Autodesk Inventor part; units mm, degrees
ref_plane "Начальная плоскость" through (0, 0, -32.5) normal (0, 0, 1) x (1, 0, 0)
ref_plane "Конечная плоскость" through (0, 0, 510.459) normal (0, 0, 1) x (1, 0, 0)
ref_plane "РабПлоскость8" through (0, 0, 510.459) normal (0, 0, 1) x (1, 0, 0)
ref_plane "Начальная плоскость" through (0, 0, -32.5) normal (0, 0, 1) x (1, 0, 0)
ref_plane "Конечная плоскость" through (0, 0, 510.459) normal (0, 0, 1) x (1, 0, 0)
sketch "Эскиз" plane through (0, 0, 0) normal (0, 0, 1) x (1, 0, 0)
  line L0 (36, -32.5) -> (0, -32.5)
  line L1 (36, -32.5) -> (36, -28.696)
  line L2 (33.6994, -26.2039) -> (9.9215, -24.3017)
  line L3 (4.4, -18.3208) -> (4.4, 18.3208)
  line L4 (33.6994, 26.2039) -> (9.9215, 24.3017)
  line L5 (36, 28.696) -> (36, 32.5)
  line L6 (0, 32.5) -> (36, 32.5)
  line L7 (0, -32.5) -> (0, 32.5)
  arc A0 (4.4, -18.3208) -> (9.9215, -24.3017) centre (10.4, -18.3208) ccw
  arc A1 (9.9215, 24.3017) -> (4.4, 18.3208) centre (10.4, 18.3208) ccw
  arc A2 (36, -28.696) -> (33.6994, -26.2039) centre (33.5, -28.696) ccw
  arc A3 (33.6994, 26.2039) -> (36, 28.696) centre (33.5, 28.696) ccw
  line L8 (0, 45.5) -> (0, -45.5) construction
  line L9 (-7.2974, 0) -> (43.7847, 0) construction
  point P0 (36, -26.388)
  point P1 (4.4, -23.86)
  point P2 (4.4, 23.86)
  point P3 (36, 26.388)
  dimension "d3" = 36
  dimension "d5" = 4.4
  dimension "d7" = 65
  dimension "d9" = 8.64
  dimension "d11" = 8.64
  dimension "d13" = 6.112
  dimension "d15" = 6.112
  dimension "d22" = 6
  dimension "d23" = 2.5
  dimension "d24" = 32.5
  dimension "d25" = 0
extrude "Тело" add sketch "Эскиз" along normal up to surface (542.959 mm away) from surface at -32.5
sketch "Sketch3" plane through (0, 0, 0) normal (0, 0, 1) x (1, 0, 0)
  line L0 (0, 0) -> (10, 0)
ref_plane "Work Plane7" through (0, 0, 0) normal (0, -1, 0) x (1, 0, 0)
sketch "Sketch4" plane through (0, 0, 0) normal (0, -1, 0) x (1, 0, 0)
  line L0 (-2, -32.5) -> (12, -32.5)
  line L1 (-2, 510.459) -> (12, 510.459)
  dimension "d29" = 542.959
ref_plane "РабПлоскость8" through (0, 0, 510.459) normal (0, 0, 1) x (1, 0, 0)
split "Разделение1" plane through (0, 0, 510.459) removes the side toward (0, 0, 1)
ref_plane "РабПлоскость9" through (18, 177.5, -32.5) normal (0, 0, -1) x (-1, 0, 0)
split "Разделение2" plane through (18, 177.5, -32.5) removes the side toward (0, 0, -1)
equation "\"d3\" = b"
equation "\"d7\" = ParH"
equation "\"d22\" = R"
equation "\"d23\" = R1"
equation "\"d24\" = 0.5 * d7"
equation "\"d16\" = G_L"
equation "\"R1\" = 2.5"
equation "\"R\" = 6"
equation "\"t1\" = 4.4"
equation "\"t2\" = 7.2"
equation "\"ParH\" = 65"
equation "\"b\" = 36"
equation "\"msp_x1\" = 0.04 * b"
equation "\"msp_x2\" = -0.08 * t1 + 0.04 * b"
equation "\"G_L\" = d29"
equation "\"ex\" = 0"
equation "\"G_OFFSET_START\" = 32.5"
equation "\"G_OFFSET_END\" = -36"
equation "\"d26\" = -G_OFFSET_START"
equation "\"d27\" = G_OFFSET_END + B_L"
equation "\"B_L\" = 546.459"
properties part number "Швеллер 6.5U-542,96 ГОСТ 8240-97"
Geometry: final body of the model. Coordinates: model frame, mm. A direction names the side the tool comes from. Coordinates: 2 decimals unless noted, no trailing zeros. Order: outer loops, then holes, each group sorted by start corner. A loop starts at its lowest first (then second) coordinate and runs counter-clockwise, first axis right, second up.
1) Draft query along Y for faces 3 (the flat face through (3, 0, 510.459)), 4 (the flat face through (21.977, 25.266, 235.179)), 5 (the flat face through (18, -32.5, 235)), 6 (the flat face through (21.977, -25.266, 235.179)). Return one class per face: released by +Y, released by -Y, zero draft, split by the parting line, or undercut.
Result sheet:
face 3: zero draft
face 4: undercut
face 5: released by -Y
face 6: undercut
2) First-contact query: P1, Ø11, axis at y = 5.5, z = 284.5, coming from the +X side; P2, Ø1.5, axis at x = 6, y = -0.5, coming from the -Z side; P3, Ø2, axis at y = 21, z = 435, coming from the +X side. Flat tips, straight axial feed; report the tip coordinate or a pass-through.
Result sheet:
P1: stops at x = 4.4
P2: passes through
P3: stops at x = 5.66
3) Section C-C (y = 9.5). Return loops of the section in (x, z), then the cut area to 3 significant figures.
Result sheet:
outline: (0, -32.5) - (4.4, -32.5) - (4.4, 510.46) - (0, 510.46) - close
area: 2,390 mm2
4) Section B-B (z = 433). Return loops of the section in (x, y), then the cut area to 3 significant figures.
Result sheet:
outline: (0, -32.5) - (36, -32.5) - (36, -28.7) arc R2.5 ccw to (33.7, -26.2) - (9.92, -24.3) arc R6 cw to (4.4, -18.32) - (4.4, 18.32) arc R6 cw to (9.92, 24.3) - (33.7, 26.2) arc R2.5 ccw to (36, 28.7) - (36, 32.5) - (0, 32.5) - close
area: 763 mm2
5) Set-up query: faces 1 (the flat face through (4.4, 0, 235)), 2 (the flat face through (3, 0, -32.5)). Return all of +Z, -Z, +X, -X, +Y, -Y with unobstructed straight access to the full face (end or side cutting, diameter ignored); none if empty.
Result sheet:
face 1: +Z, -Z, +X
face 2: -Z, +X, -X, +Y, -Y
6) Section A-A (x = 17). Return loops of the section in (y, z), then the cut area to 3 significant figures.
Result sheet:
outline: (-32.5, -32.5) - (-24.87, -32.5) - (-24.87, 510.46) - (-32.5, 510.46) - close; (24.87, -32.5) - (32.5, -32.5) - (32.5, 510.46) - (24.87, 510.46) - close
area: 8,290 mm2
7) Ray query, probe 1 along Y at (x, z) = (9.5, 21); probe 2 along X at (y, z) = (15, 26.5); probe 3 along Y at (x, z) = (14, 238.5). Return the intervals inside material, ascending.
Result sheet:
probe 1: y = -32.5 to -24.25, 24.25 to 32.5
probe 2: x = 0 to 4.4
probe 3: y = -32.5 to -24.63, 24.63 to 32.5
